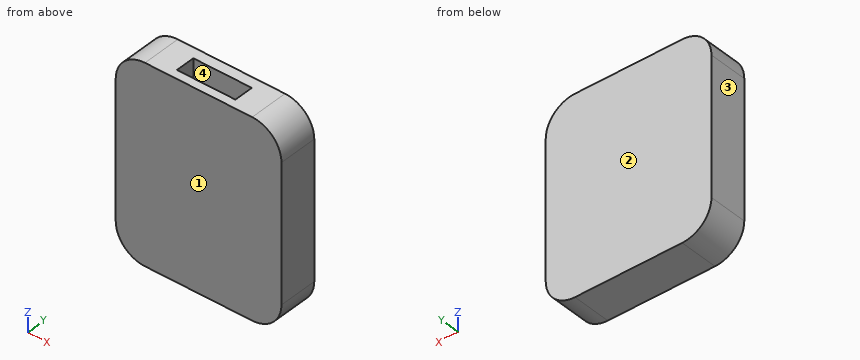
from build123d import *

# Parameters (mm, degrees)
F0_W     = 85
F0_H     = 100
F1_DEPTH = 20
F2_W     = 30
F2_H     = 10
F3_DEPTH = 20.4
F4_R     = 15


with BuildPart() as f1:
    # F0 (on Front) → F1 (new body)
    with BuildSketch(Plane.XZ):
        with Locations((4.112373, -14.619432)):
            Rectangle(F0_W, F0_H)
    extrude(amount=F1_DEPTH)

    # F2 (on face) → F3 (cut)
    with BuildSketch(Plane.XY.offset(35.380568)):
        with Locations((4.212248, -10.496597)):
            Rectangle(F2_W, F2_H)
    extrude(amount=-F3_DEPTH, mode=Mode.SUBTRACT)

    # F4
    f4_edges = [f1.edges().sort_by_distance(p)[0] for p in [
        (46.612373, -10, 35.380568),
        (-38.387627, -10, 35.380568),
        (46.612373, -10, -64.619432),
        (-38.387627, -10, -64.619432),
    ]]
    fillet(f4_edges, radius=F4_R)


solid = f1.part
Could you check a few things on this model? Use its own coordinates, in mm. Face numbers are marked on the shaded views. Coordinates: 2 decimals unless noted, no trailing zeros. Loops run counter-clockwise (first coordinate to the right, second up) from the corner with the lowest first, then second, coordinate; pieces in that order, holes last. Notation, with made-up numbers: (16.5, 41.25) -> (70.5, 41.25) arc R25 cw to (70.5, 62.25) -> close; hole circle Ø5 at (89, 87). An arc over 180 degrees is marked (long way). Answer in a Markdown table with one row per item.
(1) Imagine slicing it at A-A (y = -12). List the corners of the cut face in (x, z) for me.
Results found:
| item | result |
|---|---|
| outline | (-38.39, -49.62) arc R15 ccw to (-23.39, -64.62) -> (31.61, -64.62) arc R15 ccw to (46.61, -49.62) -> (46.61, 20.38) arc R15 ccw to (31.61, 35.38) -> (19.21, 35.38) -> (19.21, 14.98) -> (-10.79, 14.98) -> (-10.79, 35.38) -> (-23.39, 35.38) arc R15 ccw to (-38.39, 20.38) -> close |
(2) Thinking about a two-plate mould opening in Y: for the marked faces 1, 2, 3 and 4, which applies, released by +Y, released by -Y, zero draft, split by the parting line, or undercut?
Results found:
| item | result |
|---|---|
| face 1 | released by -Y |
| face 2 | released by +Y |
| face 3 | zero draft |
| face 4 | undercut |
(3) Will these pins go through, and if not, where does the flat tip stop? pin 1 Ø3 at (y, z) = (-8.5, 24.5) entering from +X; pin 2 Ø5 at (x, y) = (10, -12) entering from +Z.
Results found:
| item | result |
|---|---|
| pin 1 | stops at x = 46.38 |
| pin 2 | stops at z = 14.98 |
(4) If I drill on probe 1 along Y at (x, z) = (11.5, 28); probe 2 along X at (y, z) = (-11, 31); probe 3 along Z at (x, y) = (-30, -14.5), over which ranges is the centre line in solid material (lowest first)?
Results found:
| item | result |
|---|---|
| probe 1 | y = -20 to -15.5, -5.5 to 0 |
| probe 2 | x = -33.98 to -10.79, 19.21 to 42.21 |
| probe 3 | z = -63.08 to 33.84 |
(5) Imagine slicing it at B-B (x = 17.5). List the corners of the cut face in (y, z) for me.
Results found:
| item | result |
|---|---|
| outline | (-20, -64.62) -> (0, -64.62) -> (0, 35.38) -> (-5.5, 35.38) -> (-5.5, 14.98) -> (-15.5, 14.98) -> (-15.5, 35.38) -> (-20, 35.38) -> close |
(6) Imagine slicing it at D-D (z = -54). List the corners of the cut face in (x, y) for me, plus the area to 3 significant figures.
Results found:
| item | result |
|---|---|
| outline | (-37.73, -20) -> (45.96, -20) -> (45.96, 0) -> (-37.73, 0) -> close |
| area | 1,670 mm^2 |
(7) Imagine slicing it at C-C (y = -3). List the corners of the cut face in (x, z) for me, plus the area to 3 significant figures.
Results found:
| item | result |
|---|---|
| outline | (-38.39, -49.62) arc R15 ccw to (-23.39, -64.62) -> (31.61, -64.62) arc R15 ccw to (46.61, -49.62) -> (46.61, 20.38) arc R15 ccw to (31.61, 35.38) -> (-23.39, 35.38) arc R15 ccw to (-38.39, 20.38) -> close |
| area | 8,310 mm^2 |
